Autodesk Fusion 360 part; units mm, degrees
sketch "Sketch1" plane through (0, 0, 0) normal (0, 0, 1) x (1, 0, 0)
  circle A0 centre (0, 0) radius 25.5
  dimension "d1" = 51
extrude "Extrude1" add sketch "Sketch1" along normal blind 1.5
sketch "Sketch2" plane through (0, 0, 1.5) normal (0, 0, 1) x (-1, 0, 0)
  circle A0 centre (0, 0) radius 25.5
  circle A1 centre (0, 0) radius 17.35
  dimension "d4" = 34.7
extrude "Extrude2" add sketch "Sketch2" along normal blind 3.5 contours A1
sketch "Sketch3" plane through (0, 0, 5) normal (0, 0, 1) x (-1, 0, 0)
  circle A0 centre (0, 0) radius 17.35
  circle A1 centre (-15, 0) radius 1.25
  dimension "d8" = 2.5
  dimension "d9" = 15
extrude "Extrude3" cut sketch "Sketch3" against normal blind 20 contours A1
pattern_circular "C-Pattern1" count 10 over 360 about axis through (0, 0, 1.75) along (0, 0, 1) of "Extrude3"
sketch "Sketch4" plane through (0, 0, 5) normal (0, 0, 1) x (-1, 0, 0)
  circle A0 centre (-12.1353, 8.8168) radius 1.25
  circle A1 centre (-4.6353, 14.2658) radius 1.25
  circle A2 centre (4.6353, 14.2658) radius 1.25
  circle A3 centre (12.1353, 8.8168) radius 1.25
  circle A4 centre (15, 0) radius 1.25
  circle A5 centre (12.1353, -8.8168) radius 1.25
  circle A6 centre (4.6353, -14.2658) radius 1.25
  circle A7 centre (-4.6353, -14.2658) radius 1.25
  circle A8 centre (-12.1353, -8.8168) radius 1.25
  circle A9 centre (-15, 0) radius 1.25
  circle A10 centre (0, 0) radius 17.35
  circle A11 centre (0, 0) radius 8
  dimension "d14" = 16
extrude "Extrude4" cut sketch "Sketch4" against normal blind 20 contours A11
chamfer "Chamfer1" distance 1 angle 45 1 edges at (7.4586, -2.8929, 5)
sketch "Sketch5" plane through (0, 0, 5) normal (0, 0, 1) x (-1, 0, 0)
  circle A0 centre (0, 0) radius 17.35
  circle A1 centre (-15, 0) radius 1.25
  circle A2 centre (-12.1353, -8.8168) radius 1.25
  circle A3 centre (-4.6353, -14.2658) radius 1.25
  circle A4 centre (4.6353, -14.2658) radius 1.25
  circle A5 centre (12.1353, -8.8168) radius 1.25
  circle A6 centre (15, 0) radius 1.25
  circle A7 centre (12.1353, 8.8168) radius 1.25
  circle A8 centre (4.6353, 14.2658) radius 1.25
  circle A9 centre (-4.6353, 14.2658) radius 1.25
  circle A10 centre (-12.1353, 8.8168) radius 1.25
  circle A11 centre (0, 0) radius 9
equation "d4 = 35 mm - offset"
equation "offset = 0.3 mm"
Part model, mm, in its own coordinate system. A direction names the side the tool comes from. Round coordinates to 2 decimals unless told otherwise and drop trailing zeros. Loops run counter-clockwise (first coordinate to the right, second up) from the corner with the lowest first, then second, coordinate; pieces in that order, holes last.
1. Slice it at B-B (y = 0). Give the cut face in (x, z), and give its area (4 significant figures).
Solutions:
outline: (-25.5, 0) - (-16.25, 0) - (-16.25, 5) - (-17.35, 5) - (-17.35, 1.5) - (-25.5, 1.5) - close; (-13.75, 0) - (-8, 0) - (-8, 4) - (-9, 5) - (-13.75, 5) - close; (8, 0) - (13.75, 0) - (13.75, 5) - (9, 5) - (8, 4) - close; (16.25, 0) - (25.5, 0) - (25.5, 1.5) - (17.35, 1.5) - (17.35, 5) - (16.25, 5) - close
area: 91.95 mm2
2. Drill centre lines: line 1 along Y through (x, z) = (-5, 3.9) (3 decimals); line 2 along Y through (x, z) = (5.5, 4.7); line 3 along X through (y, z) = (6.5, 1.3). Where is each one in solid material? Low to high.
Solutions:
line 1: y = -16.614 to -15.461, -13.07 to -6.245, 6.245 to 13.07, 15.461 to 16.614
line 2: y = -16.46 to -15.17, -13.36 to -6.74, 6.74 to 13.36, 15.17 to 16.46
line 3: x = -24.66 to -4.66, 4.66 to 24.66
3. Two-plate mould, pull along Y, no slides. Class faces 3 (the face through (-6, 6, 0)), 4 (the face through (2.259, 17.202, 3.226)), 5 (the face through (16.25, -0.05, 2.54)): pulls with the +Y half, pulls with the -Y half, needs draft (parallel to the pull), parting line crosses it, or undercut.
Solutions:
face 3: needs draft
face 4: parting line crosses it
face 5: undercut
4. 3-axis set-ups, long thin cutter, end or side, ignore diameter. For faces 1 (the face through (-4.624, -13.016, 2.535)), 2 (the face through (17, -5, 1.5)): which of +Z, -Z, +X, -X, +Y, -Y reach the whole face in a straight line?
Solutions:
face 1: +Z, -Z
face 2: +Z
5. Flat gauge pins, fed straight in: pin 1 (1 mm diameter, centred on x = 18, z = 0.5, fed in from +Y); pin 2 (2 mm diameter, centred on y = -9, z = 1, fed in from -X). Where does each tip first touch, or does it go through?
Solutions:
pin 1: stops at y = 18.55
pin 2: stops at x = -24.21
6. Slice it at A-A (x = 0). Give the cut face in (y, z).
Solutions:
outline: (-25.5, 0) - (-8, 0) - (-8, 4) - (-9, 5) - (-17.35, 5) - (-17.35, 1.5) - (-25.5, 1.5) - close; (8, 0) - (25.5, 0) - (25.5, 1.5) - (17.35, 1.5) - (17.35, 5) - (9, 5) - (8, 4) - close
7. Slice it at D-D (x = -15). Give the cut face in (y, z), and give its area (3 significant figures).
Solutions:
outline: (-20.62, 0) - (-1.25, 0) - (-1.25, 5) - (-8.72, 5) - (-8.72, 1.5) - (-20.62, 1.5) - close; (1.25, 0) - (20.62, 0) - (20.62, 1.5) - (8.72, 1.5) - (8.72, 5) - (1.25, 5) - close
area: 110 mm2
